Geometry: final body of the model. Coordinates: model frame, mm. Give positions to 0.01 mm unless a question says otherwise; leave off trailing zeros. Write each loop counter-clockwise with the first axis right and the second up, starting at its lowest first coordinate (ties: lowest second). Pieces come first, ordered by that corner, then holes. Notation, with made-up numbers: (35.5, 40.5) -> (41.5, 40.5) arc R25 cw to (41.5, 70.5) -> close; hole circle Ø3 at (1.5, 75). An arc over 180 degrees is marked (long way). Use CSV: the item, a comma, the result in double quotes. Start each with the question number.
1) Section C-C (y = 3.95). Output: boundary loops of the cut face in (x, z).
2) Section A-A (z = 0). Output: boundary loops of the cut face in (x, y), plus the area to 3 significant figures.
3) Section B-B (x = -21). Output: boundary loops of the cut face in (y, z), plus the area to 3 significant figures.
4) Draft query along X for faces 1 (the face through (-19.82, 2.35, -1.08)), 2 (the face through (0, 2, 6.751)), 3 (the face through (26.817, 2.348, -0.148)). Return one class per face: pulls with the +X half, pulls with the -X half, needs draft (parallel to the pull), parting line crosses it, or undercut.
5) Material intervals for line 1 (Z direction, x = 0, y = 3); line 2 (X direction, y = 0.8, z = 1.25); line 3 (Z direction, x = 21, y = 1.2), sorted ascending. Write a range as [from, to].
6) Section D-D (x = 21). Output: boundary loops of the cut face in (y, z).
```python
from build123d import *

# Parameters (mm, degrees)
BOSS_EXTRUDE1_DEPTH      = 4.763
M3_CLEARANCE_HOLE1_D     = 3.2
M3_CLEARANCE_HOLE1_DEPTH = 4.763


with BuildPart() as part:
    # Sketch1 → Boss-Extrude1 (new body)
    with BuildSketch(Plane(origin=(0, 0, 0), x_dir=(1, 0, 0), z_dir=(0, 1, 0))):
        with BuildLine():
            Line((-19.932225786, 6.750936854), (20.067774214, 6.750936854))
            ThreePointArc((20.067774214, 6.750936854), (26.818711069, 0), (20.067774214, -6.750936854))
            Line((20.067774214, -6.750936854), (-19.932225786, -6.750936854))
            ThreePointArc((-19.932225786, -6.750936854), (-26.68316264, 0), (-19.932225786, 6.750936854))
        make_face()
    extrude(amount=BOSS_EXTRUDE1_DEPTH)

    # M3 Clearance Hole1
    with Locations(Plane(origin=(0, 4.763, 0), x_dir=(1, 0, 0), z_dir=(0, 1, 0))):
        with Locations((-21, 0), (0, 0), (21, 0)):
            Hole(M3_CLEARANCE_HOLE1_D / 2, depth=M3_CLEARANCE_HOLE1_DEPTH)


solid = part.part
```
Answers follow:
1,outline,"(-19.93, -6.75) -> (20.07, -6.75) arc R6.75 ccw to (20.07, 6.75) -> (-19.93, 6.75) arc R6.75 ccw to start; hole circle Ø3.2 at (-21, 0); hole circle Ø3.2 at (0, 0); hole circle Ø3.2 at (21, 0)"
2,outline,"(-26.68, 0) -> (-22.6, 0) -> (-22.6, 4.76) -> (-26.68, 4.76) -> close; (-19.4, 0) -> (-1.6, 0) -> (-1.6, 4.76) -> (-19.4, 4.76) -> close; (1.6, 0) -> (19.4, 0) -> (19.4, 4.76) -> (1.6, 4.76) -> close; (22.6, 0) -> (26.82, 0) -> (26.82, 4.76) -> (22.6, 4.76) -> close"
2,area,"209 mm^2"
3,outline,"(0, -6.67) -> (4.76, -6.67) -> (4.76, -1.6) -> (0, -1.6) -> close; (0, 1.6) -> (4.76, 1.6) -> (4.76, 6.67) -> (0, 6.67) -> close"
3,area,"48.3 mm^2"
4,face 1,"undercut"
4,face 2,"needs draft"
4,face 3,"pulls with the +X half"
5,line 1,"z = [-6.75, -1.6], [1.6, 6.75]"
5,line 2,"x = [-26.57, -22], [-20, -1], [1, 20], [22, 26.7]"
5,line 3,"z = [-6.69, -1.6], [1.6, 6.69]"
6,outline,"(0, -6.69) -> (4.76, -6.69) -> (4.76, -1.6) -> (0, -1.6) -> close; (0, 1.6) -> (4.76, 1.6) -> (4.76, 6.69) -> (0, 6.69) -> close"
